For this review, take the finished solid that the model builds, in its own axes (mm). A direction names the side the tool comes from. Coordinates: 2 decimals unless noted, no trailing zeros. Loops run counter-clockwise (first coordinate to the right, second up) from the corner with the lowest first, then second, coordinate; pieces in that order, holes last.
```python
from build123d import *

# Parameters (mm, degrees)
SKETCH1_R           = 50.546
BOSS_EXTRUDE1_DEPTH = 6.35
SKETCH3_W           = 6.35
SKETCH3_H           = 94.144269948
BOSS_EXTRUDE2_DEPTH = 203.2
BOSS_EXTRUDE3_DEPTH = 6.35
CUT_EXTRUDE1_REACH  = 229.426
SKETCH5_R           = 6.35
SKETCH7_R           = 3.175
BOSS_EXTRUDE4_DEPTH = 215.9
SKETCH8_R           = 1.27
CUT_EXTRUDE2_DEPTH  = 237.368563766
SKETCH9_W           = 3.175
SKETCH9_H           = 76.2
BOSS_EXTRUDE5_DEPTH = 19.05
SKETCH10_W          = 19.05
SKETCH10_H          = 2.54
BOSS_EXTRUDE6_DEPTH = 25.4
CUT_EXTRUDE3_REACH  = 203.094
SKETCH11_R          = 1.27
SKETCH12_W          = 17.48
SKETCH12_H          = 27.88
SKETCH12_W_2        = 12.4
SKETCH12_H_2        = 22.8
BOSS_EXTRUDE7_DEPTH = 18.3
SKETCH13_R          = 3.81
SKETCH13_R_2        = 1.27
BOSS_EXTRUDE8_DEPTH = 5.08


with BuildPart() as part:
    # Sketch1 → Boss-Extrude1 (new body)
    with BuildSketch(Plane(origin=(0, 0, 0), x_dir=(1, 0, 0), z_dir=(0, 1, 0))):
        with Locations(Location((0, 0, 0), (0, 0, 270))):
            Circle(SKETCH1_R)
    extrude(amount=BOSS_EXTRUDE1_DEPTH)

    # Sketch3 → Boss-Extrude2 (add)
    with BuildSketch(Plane(origin=(0, 6.35, 0), x_dir=(1, 0, 0), z_dir=(0, 1, 0))):
        with Locations((15.24, 0)):
            Rectangle(SKETCH3_W, SKETCH3_H)
    extrude(amount=BOSS_EXTRUDE2_DEPTH)

    # Sketch4 → Boss-Extrude3 (add)
    with BuildSketch(Plane(origin=(0, 209.55, 0), x_dir=(1, 0, 0), z_dir=(0, 1, 0))):
        with BuildLine():
            ThreePointArc((18.415, 47.072134974), (-50.546, 0), (18.415, -47.072134974))
            ThreePointArc((18.415, -47.072134974), (50.546, 0), (18.415, 47.072134974))
        make_face()
    extrude(amount=BOSS_EXTRUDE3_DEPTH)

    # Sketch5 → Cut-Extrude1 (cut, up to next)
    with BuildSketch(Plane(origin=(0, 215.9, 0), x_dir=(1, 0, 0), z_dir=(0, 1, 0)), mode=Mode.PRIVATE) as cut_extrude1_sk1:
        with Locations(Location((0, 0, 0), (0, 0, 270))):
            Circle(SKETCH5_R)
    cut_extrude1_tool1 = extrude(cut_extrude1_sk1.sketch, amount=-CUT_EXTRUDE1_REACH, mode=Mode.PRIVATE) & part.part
    add(cut_extrude1_tool1.solids().sort_by_distance((0, 215.9, 0))[0], mode=Mode.SUBTRACT)

    # Sketch7 → Boss-Extrude4 (add)
    with BuildSketch(Plane(origin=(0, 6.35, 0), x_dir=(1, 0, 0), z_dir=(0, 1, 0))):
        with Locations(Location((0, 0, 0), (0, 0, 270))):
            Circle(SKETCH7_R)
    extrude(amount=BOSS_EXTRUDE4_DEPTH)

    # Sketch8 → Cut-Extrude2 (cut, through all)
    with BuildSketch(Plane.ZY.offset(-12.065)):
        with Locations((-19.05, 69.85)):
            Circle(SKETCH8_R)
    extrude(amount=-CUT_EXTRUDE2_DEPTH, mode=Mode.SUBTRACT)

    # Sketch9 → Boss-Extrude5 (add)
    with BuildSketch(Plane.ZY.offset(-12.065)):
        with Locations((-45.484634974, 69.85)):
            Rectangle(SKETCH9_W, SKETCH9_H)
    extrude(amount=BOSS_EXTRUDE5_DEPTH)

    # Sketch10 → Boss-Extrude6 (add)
    with BuildSketch(Plane.XY.offset(-43.897134974)):
        with Locations((2.54, 33.02)):
            Rectangle(SKETCH10_W, SKETCH10_H)
    extrude(amount=BOSS_EXTRUDE6_DEPTH)

    # Sketch11 → Cut-Extrude3 (cut, up to next)
    with BuildSketch(Plane(origin=(0, 34.29, 0), x_dir=(1, 0, 0), z_dir=(0, 1, 0)), mode=Mode.PRIVATE) as cut_extrude3_sk1:
        with Locations(Location((-1.905, 36.312665469, 0), (0, 0, 180))):
            Circle(SKETCH11_R)
    cut_extrude3_tool1 = extrude(cut_extrude3_sk1.sketch, amount=-CUT_EXTRUDE3_REACH, mode=Mode.PRIVATE) & part.part
    add(cut_extrude3_tool1.solids().sort_by_distance((-1.905, 34.29, -36.312665))[0], mode=Mode.SUBTRACT)

    # Sketch12 → Boss-Extrude7 (add)
    with BuildSketch(Plane.ZY.offset(-12.065)):
        with Locations((23.352648963, 74.888693437)):
            Rectangle(SKETCH12_W, SKETCH12_H)
        with Locations((23.352648963, 74.888693437)):
            Rectangle(SKETCH12_W_2, SKETCH12_H_2, mode=Mode.SUBTRACT)
    extrude(amount=BOSS_EXTRUDE7_DEPTH)

    # Sketch13 → Boss-Extrude8 (add)
    # profile 1 of 4: a face of its own
    with BuildSketch(Plane(origin=(18.415, 0, 0), x_dir=(0, 0, -1), z_dir=(1, 0, 0))):
        with Locations(Location((-38.1, 158.75, 0), (0, 0, 180))):
            Circle(SKETCH13_R)
        with Locations((-38.1, 158.75)):
            Circle(SKETCH13_R_2, mode=Mode.SUBTRACT)
    # profile 2 of 4: a face of its own
    with BuildSketch(Plane(origin=(18.415, 0, 0), x_dir=(0, 0, -1), z_dir=(1, 0, 0))):
        with Locations(Location((38.1, 158.75, 0), (0, 0, 180))):
            Circle(SKETCH13_R)
        with Locations((38.1, 158.75)):
            Circle(SKETCH13_R_2, mode=Mode.SUBTRACT)
    # profile 3 of 4: a face of its own
    with BuildSketch(Plane(origin=(18.415, 0, 0), x_dir=(0, 0, -1), z_dir=(1, 0, 0))):
        with Locations(Location((-38.1, 57.15, 0), (0, 0, 180))):
            Circle(SKETCH13_R)
        with Locations((-38.1, 57.15)):
            Circle(SKETCH13_R_2, mode=Mode.SUBTRACT)
    # profile 4 of 4: a face of its own
    with BuildSketch(Plane(origin=(18.415, 0, 0), x_dir=(0, 0, -1), z_dir=(1, 0, 0))):
        with Locations(Location((38.1, 57.15, 0), (0, 0, 180))):
            Circle(SKETCH13_R)
        with Locations((38.1, 57.15)):
            Circle(SKETCH13_R_2, mode=Mode.SUBTRACT)
    extrude(amount=BOSS_EXTRUDE8_DEPTH)


solid = part.part
```
Q1. Consider section B-B (y = 136.5). State the section outline as (x, z) points (3 decimals).
Q2. The part is to be moulded in two halves that separate along Z. For faces 1 (the face through (3, 75, 17.153)), 2 (the face through (15, 107, 47.072)), 3 (the face through (2, 31.75, -33)), say which applies: +Z half, -Z half, draft (parallel to the pull), parting line (faces both ways), or undercut.
Q3. Consider section D-D (z = 24.5). State the section outline as (x, y) points (3 decimals).
Q4. Machinability: for faces 4 (the face through (20.92, 58.61, -34.58)), 5 (the face through (23.495, 159, 40)), 6 (the face through (3, 60.949, 23)), which of the approach directions +Z, -Z, +X, -X, +Y, -Y give a long, thin tool a straight path to every point of the face, cutting with its end or side? Answer none if there is none.
Q5. Consider section A-A (z = 0). State the section outline as (x, y) points (3 decimals).
Q6. Consider section C-C (x = 33). State the section outline as (y, z) points, then the cut area to 3 significant figures.
Q7. For pin 1 Ø8.5 at (y, z) = (58.5, -39) entering from +X (3 decimals); pin 2 Ø2 at (x, y) = (15.5, 117.5) entering from +Z; pin 3 Ø12.5 at (x, y) = (4, 95.5) entering from -Z; pin 4 Ø21 at (x, z) = (-1, -26.5) entering from -Y, all flat-tipped, find the tip position at first contact; note any pin that passes through.
Q8. Wall thickness on probe 1 along Y at (x, z) = (21, 38); probe 2 along Z at (x, y) = (22.3, 158.75); probe 3 along Y at (x, z) = (-14, -8.5): over which ranges is each line inside the solid? List them lowest first.
Model answer:
1. outline: circle Ø6.35 at (0, 0); (12.065, -47.072) - (18.415, -47.072) - (18.415, 47.072) - (12.065, 47.072) - close
2. face 1: undercut
2. face 2: +Z half
2. face 3: draft
3. outline: (-44.211, 0) - (44.211, 0) - (44.211, 6.35) - (18.415, 6.35) - (18.415, 209.55) - (44.211, 209.55) - (44.211, 215.9) - (-44.211, 215.9) - (-44.211, 209.55) - (12.065, 209.55) - (12.065, 88.829) - (-6.235, 88.829) - (-6.235, 86.289) - (12.065, 86.289) - (12.065, 63.489) - (-6.235, 63.489) - (-6.235, 60.949) - (12.065, 60.949) - (12.065, 6.35) - (-44.211, 6.35) - close
4. face 4: +X
4. face 5: +Z, -Z, +X
4. face 6: +Z, -X
5. outline: (-50.546, 0) - (50.546, 0) - (50.546, 6.35) - (18.415, 6.35) - (18.415, 209.55) - (50.546, 209.55) - (50.546, 215.9) - (6.35, 215.9) - (6.35, 209.55) - (12.065, 209.55) - (12.065, 6.35) - (3.175, 6.35) - (3.175, 222.25) - (-3.175, 222.25) - (-3.175, 6.35) - (-50.546, 6.35) - close; (-50.546, 209.55) - (-6.35, 209.55) - (-6.35, 215.9) - (-50.546, 215.9) - close
6. outline: (0, -38.29) - (6.35, -38.29) - (6.35, 38.29) - (0, 38.29) - close; (209.55, -38.29) - (215.9, -38.29) - (215.9, 38.29) - (209.55, 38.29) - close
6. area: 972 mm2
7. pin 1: stops at x = 23.495
7. pin 2: stops at z = 47.07
7. pin 3: stops at z = -47.07
7. pin 4: stops at y = 0
8. probe 1: y = 0 to 6.35, 53.34 to 55.88, 58.42 to 60.96, 154.94 to 157.48, 160.02 to 162.56, 209.55 to 215.9
8. probe 2: z = -41.91 to -39.37, -36.83 to -34.29, 34.29 to 36.83, 39.37 to 41.91
8. probe 3: y = 0 to 6.35, 209.55 to 215.9
